```python
from build123d import *

# Parameters (mm, degrees)
F0_R     = 14.2875
F1_DEPTH = 25.4
F2_DEPTH = 50.8


with BuildPart() as f1:
    # F0 (on Front) → F1 (new body)
    with BuildSketch(Plane.XZ):
        with BuildLine():
            ThreePointArc((5.0235075245, -28.1299661776), (21.9097849432, -18.3437168737), (28.575, 0))
            ThreePointArc((28.575, 0), (23.3127267057, 16.5241459249), (9.4640709678, 26.9622325803))
            Line((9.4640709678, 26.9622325803), (0, 28.575))
            ThreePointArc((0, 28.575), (-28.4635241012, -2.5215909141), (5.0235075245, -28.1299661776))
        make_face()
        with BuildLine():
            ThreePointArc((-13.4703841816, 4.7625), (0, 14.2875), (13.4703841816, 4.7625))
            Line((13.4703841816, 4.7625), (19.3582428957, 4.7625))
            Line((19.3582428957, 4.7625), (19.3582428957, -4.7625))
            Line((19.3582428957, -4.7625), (13.4703841816, -4.7625))
            ThreePointArc((13.4703841816, -4.7625), (0, -14.2875), (-13.4703841816, -4.7625))
            Line((-13.4703841816, -4.7625), (-18.7417571043, -4.7625))
            Line((-18.7417571043, -4.7625), (-18.7417571043, 4.7625))
            Line((-18.7417571043, 4.7625), (-13.4703841816, 4.7625))
        make_face(mode=Mode.SUBTRACT)
        with BuildLine():
            ThreePointArc((9.4640709678, 26.9622325803), (23.3127267057, 16.5241459249), (28.575, 0))
            ThreePointArc((28.575, 0), (21.9097849432, -18.3437168737), (5.0235075245, -28.1299661776))
            Line((5.0235075245, -28.1299661776), (56.8131846517, -18.881257763))
            ThreePointArc((56.8131846517, -18.881257763), (35.2362588947, 0.3389697117), (57.4834105655, 18.7792818522))
            Line((57.4834105655, 18.7792818522), (9.4640709678, 26.9622325803))
        make_face()
        with BuildLine():
            Line((0, 28.575), (9.4640709678, 26.9622325803))
            ThreePointArc((9.4640709678, 26.9622325803), (4.8002515047, 28.1689227783), (0, 28.575))
        make_face()
        with BuildLine():
            ThreePointArc((73.3332428957, 0), (68.84115645, 12.2869708612), (57.4834105655, 18.7792818522))
            ThreePointArc((57.4834105655, 18.7792818522), (35.2362588947, 0.3389697117), (56.8131846517, -18.881257763))
            ThreePointArc((56.8131846517, -18.881257763), (68.6202211417, -12.5440645237), (73.3332428957, 0))
        make_face()
        with Locations((54.2832428957, 0)):
            Circle(F0_R, mode=Mode.SUBTRACT)
    extrude(amount=F1_DEPTH)

    # F0 (on Front) → F2 (join)
    with BuildSketch(Plane.XZ):
        with BuildLine():
            ThreePointArc((5.0235075245, -28.1299661776), (21.9097849432, -18.3437168737), (28.575, 0))
            ThreePointArc((28.575, 0), (23.3127267057, 16.5241459249), (9.4640709678, 26.9622325803))
            Line((9.4640709678, 26.9622325803), (0, 28.575))
            ThreePointArc((0, 28.575), (-28.4635241012, -2.5215909141), (5.0235075245, -28.1299661776))
        make_face()
        with BuildLine():
            ThreePointArc((-13.4703841816, 4.7625), (0, 14.2875), (13.4703841816, 4.7625))
            Line((13.4703841816, 4.7625), (19.3582428957, 4.7625))
            Line((19.3582428957, 4.7625), (19.3582428957, -4.7625))
            Line((19.3582428957, -4.7625), (13.4703841816, -4.7625))
            ThreePointArc((13.4703841816, -4.7625), (0, -14.2875), (-13.4703841816, -4.7625))
            Line((-13.4703841816, -4.7625), (-18.7417571043, -4.7625))
            Line((-18.7417571043, -4.7625), (-18.7417571043, 4.7625))
            Line((-18.7417571043, 4.7625), (-13.4703841816, 4.7625))
        make_face(mode=Mode.SUBTRACT)
        with BuildLine():
            ThreePointArc((-13.4703841816, -4.7625), (-14.2875, 0), (-13.4703841816, 4.7625))
            Line((-13.4703841816, 4.7625), (-18.7417571043, 4.7625))
            Line((-18.7417571043, 4.7625), (-18.7417571043, -4.7625))
            Line((-18.7417571043, -4.7625), (-13.4703841816, -4.7625))
        make_face()
    extrude(amount=F2_DEPTH)


solid = f1.part
```
Build history of the part. All positions in model axes, mm. A direction names the side the tool comes from. Round coordinates to 2 decimals unless told otherwise and drop trailing zeros. Order: outer loops, then holes, each group sorted by start corner. A loop starts at its lowest first (then second) coordinate and runs counter-clockwise, first axis right, second up. Notation, with made-up numbers: (10.25, 4) - (63.25, 4) arc R5 cw to (63.25, 11) - close; hole circle Ø3 at (-19.75, -11.5). An arc over 180 degrees is marked (long way). Use a Markdown table: item, result.
1) Saw through at C-C on z = -6.5. Write the cut outline in (x, y), and give its area (3 significant figures).
Recorded:
| item | result |
|---|---|
| outline | (-27.83, -50.8) - (-12.72, -50.8) - (-12.72, 0) - (-27.83, 0) - close; (12.72, -50.8) - (27.83, -50.8) - (27.83, -25.4) - (41.56, -25.4) - (41.56, 0) - (12.72, 0) - close; (67.01, -25.4) - (72.19, -25.4) - (72.19, 0) - (67.01, 0) - close |
| area | 2,010 mm² |
2) Saw through at B-B on x = 46. Write the cut outline in (y, z), and give its area (3 significant figures).
Recorded:
| item | result |
|---|---|
| outline | (-25.4, -20.81) - (0, -20.81) - (0, -11.64) - (-25.4, -11.64) - close; (-25.4, 11.64) - (0, 11.64) - (0, 20.74) - (-25.4, 20.74) - close |
| area | 464 mm² |
3) Saw through at A-A on y = -9. Give the number of separate pieces and of enclosed holes in the cut face, and give its area (3 significant figures).
Recorded:
| item | result |
|---|---|
| separate pieces | 1 |
| enclosed holes | 2 |
| area | 3,130 mm² |
4) Tool access for faces 4 (the face through (4.798, -37.922, 27.757)), 5 (the face through (16, -25, -4.762)), 6 (the face through (-13, -50.8, 7)): list every direction of +Z, -Z, +X, -X, +Y, -Y with a clear straight run to the whole face (end or side of a thin tool).
Recorded:
| item | result |
|---|---|
| face 4 | +Z, +X, -Y |
| face 5 | +Y, -Y |
| face 6 | +Z, -Z, +X, -X, -Y |
5) Pull direction Z, two halves, no side cores. Call faces 1 (the face through (33.81, -12.522, 22.813)), 2 (the face through (30.56, -12.52, -23.57)), 3 (the face through (16, -25, 4.762)): pulls with the +Z half, pulls with the -Z half, needs draft (parallel to the pull), parting line crosses it, or undercut.
Recorded:
| item | result |
|---|---|
| face 1 | pulls with the +Z half |
| face 2 | pulls with the -Z half |
| face 3 | undercut |
6) Wall check: L1, parallel to X at y = -19, z = -8; L2, parallel to Z at x = 0, y = -28 (1 decimal); L3, parallel to Y at x = 41, z = -13.5. Give the ranges that are in metal, low to high.
Recorded:
| item | result |
|---|---|
| L1 | x = -27.43 to -11.84, 11.84 to 42.45, 66.12 to 71.57 |
| L2 | z = -28.6 to -14.3, 14.3 to 28.6 |
| L3 | y = -25.4 to 0 |
7) Flat gauge pins, fed straight in: pin 1 Ø12 at (y, z) = (-30, -6) entering from +X; pin 2 Ø1.8 at (x, y) = (16, -26.5) entering from +Z; pin 3 Ø1.8 at (x, y) = (16.5, -16) entering from -Z. Where does each tip first touch, or does it go through?
Recorded:
| item | result |
|---|---|
| pin 1 | stops at x = 73.21 |
| pin 2 | stops at z = 24.26 |
| pin 3 | stops at z = -26.24 |
